```python
from build123d import *
from build123d.topology import SkipClean

# Parameters (mm, degrees)
CROQUIS1_R                      = 1.6
CROQUIS1_R_2                    = 2.75
SALIENTE_EXTRUIR1_DEPTH         = 1.5
SALIENTE_EXTRUIR3_START         = 15.1
CROQUIS3_R                      = 4
SALIENTE_EXTRUIR3_DEPTH         = 15.1
CROQUIS4_R                      = 3.1
CORTAR_EXTRUIR1_DEPTH           = 7.87
SALIENTE_EXTRUIR4_START         = -0.85
CROQUIS4_3_R                    = 3.1
CROQUIS4_3_R_2                  = 2.5
SALIENTE_EXTRUIR4_DEPTH         = 6.17
CROQUIS5_R                      = 2.5
CORTAR_EXTRUIR3_DEPTH           = 1.5
CORTAR_EXTRUIR3_DRAFT           = -17
CORTAR_EXTRUIR3_PROFILE_2_DEPTH = 1.5
CORTAR_EXTRUIR3_PROFILE_2_DRAFT = -17
CORTAR_EXTRUIR3_PROFILE_3_DEPTH = 1.5
CORTAR_EXTRUIR3_PROFILE_3_DRAFT = -17
CORTAR_EXTRUIR3_PROFILE_4_DEPTH = 1.5
CORTAR_EXTRUIR3_PROFILE_4_DRAFT = -17
NERVIO1_REACH                   = 45.809
CROQUIS6_WALL_W                 = 105.302560272
CROQUIS6_WALL_H                 = 3


with BuildPart() as part:
    # Croquis1 → Saliente-Extruir1 (new body)
    with BuildSketch(Plane(origin=(0, 0, 0), x_dir=(1, 0, 0), z_dir=(0, 1, 0))):
        with BuildLine():
            Line((-0.802944128, 3.918581469), (27.882639679, 9.796453672))
            ThreePointArc((27.882639679, 9.796453672), (39.89, 0), (27.882639679, -9.796453672))
            Line((27.882639679, -9.796453672), (-0.802944128, -3.918581469))
            ThreePointArc((-0.802944128, -3.918581469), (-4, 0), (-0.802944128, 3.918581469))
        make_face()
        with Locations(Location((29.89, 7, 0), (0, 0, 270))):
            Circle(CROQUIS1_R, mode=Mode.SUBTRACT)
        with Locations(Location((36.89, 0, 0), (0, 0, 270))):
            Circle(CROQUIS1_R, mode=Mode.SUBTRACT)
        with Locations(Location((29.89, -7, 0), (0, 0, 270))):
            Circle(CROQUIS1_R, mode=Mode.SUBTRACT)
        with Locations(Location((22.89, 0, 0), (0, 0, 270))):
            Circle(CROQUIS1_R, mode=Mode.SUBTRACT)
        with Locations(Location((29.89, 0, 0), (0, 0, 270))):
            Circle(CROQUIS1_R_2, mode=Mode.SUBTRACT)
    extrude(amount=SALIENTE_EXTRUIR1_DEPTH)

    # Croquis3 → Saliente-Extruir3 (add)
    with SkipClean():  # the faces are left unmerged after this step: merging them gives an invalid solid
        with BuildSketch(Plane.XZ.offset(SALIENTE_EXTRUIR3_START)):
            with Locations(Location((0, 0, 0), (0, 0, 258.419996521))):
                Circle(CROQUIS3_R)
        extrude(amount=-SALIENTE_EXTRUIR3_DEPTH)

    # Croquis4 → Cortar-Extruir1 (cut)
    with SkipClean():  # the faces are left unmerged after this step: merging them gives an invalid solid
        with BuildSketch(Plane.XZ.offset(15.1)):
            with Locations(Location((0, 0, 0), (0, 0, 270))):
                Circle(CROQUIS4_R)
        extrude(amount=-CORTAR_EXTRUIR1_DEPTH, mode=Mode.SUBTRACT)

    # Croquis4<3> → Saliente-Extruir4 (add)
    with SkipClean():  # the faces are left unmerged after this step: merging them gives an invalid solid
        with BuildSketch(Plane.XZ.offset(15.1).offset(SALIENTE_EXTRUIR4_START)):
            with Locations(Location((0, 0, 0), (0, 0, 270))):
                Circle(CROQUIS4_3_R)
            with Locations(Location((0, 0, 0), (0, 0, 270))):
                Circle(CROQUIS4_3_R_2, mode=Mode.SUBTRACT)
        extrude(amount=-SALIENTE_EXTRUIR4_DEPTH)


with BuildPart() as cortar_extruir3_tool:
    # Croquis5 → Cortar-Extruir3 (with draft: the straight prism first)
    with BuildSketch(Plane(origin=(0, 1.5, 0), x_dir=(1, 0, 0), z_dir=(0, 1, 0))):
        with Locations((29.89, 7)):
            Circle(CROQUIS5_R)
    extrude(amount=-CORTAR_EXTRUIR3_DEPTH)
    # Cortar-Extruir3: the draft: its side faces are tilted about the plane it starts from
    cortar_extruir3_sides = [cortar_extruir3_tool.faces().sort_by_distance(p)[0] for p in [
        (27.39, 0.75, -7),
    ]]
    draft(cortar_extruir3_sides, Plane(origin=(0, 1.5, 0), x_dir=(1, 0, 0), z_dir=(0, 1, 0)), CORTAR_EXTRUIR3_DRAFT)


with BuildPart() as part_1:
    add(part.part)

    # Cortar-Extruir3: cut by cortar_extruir3_tool
    add(cortar_extruir3_tool.part, mode=Mode.SUBTRACT)


with BuildPart() as cortar_extruir3_profile_2_tool:
    # Croquis5 → Cortar-Extruir3 profile 2 (with draft: the straight prism first)
    with BuildSketch(Plane(origin=(0, 1.5, 0), x_dir=(1, 0, 0), z_dir=(0, 1, 0))):
        with Locations((36.89, 0)):
            Circle(CROQUIS5_R)
    extrude(amount=-CORTAR_EXTRUIR3_PROFILE_2_DEPTH)
    # Cortar-Extruir3 profile 2: the draft: its side faces are tilted about the plane it starts from
    cortar_extruir3_profile_2_sides = [cortar_extruir3_profile_2_tool.faces().sort_by_distance(p)[0] for p in [
        (34.39, 0.75, 0),
    ]]
    draft(cortar_extruir3_profile_2_sides, Plane(origin=(0, 1.5, 0), x_dir=(1, 0, 0), z_dir=(0, 1, 0)), CORTAR_EXTRUIR3_PROFILE_2_DRAFT)


with BuildPart() as part_2:
    add(part_1.part)

    # Cortar-Extruir3 profile 2: cut by cortar_extruir3_profile_2_tool
    add(cortar_extruir3_profile_2_tool.part, mode=Mode.SUBTRACT)


with BuildPart() as cortar_extruir3_profile_3_tool:
    # Croquis5 → Cortar-Extruir3 profile 3 (with draft: the straight prism first)
    with BuildSketch(Plane(origin=(0, 1.5, 0), x_dir=(1, 0, 0), z_dir=(0, 1, 0))):
        with Locations((29.89, -7)):
            Circle(CROQUIS5_R)
    extrude(amount=-CORTAR_EXTRUIR3_PROFILE_3_DEPTH)
    # Cortar-Extruir3 profile 3: the draft: its side faces are tilted about the plane it starts from
    cortar_extruir3_profile_3_sides = [cortar_extruir3_profile_3_tool.faces().sort_by_distance(p)[0] for p in [
        (27.39, 0.75, 7),
    ]]
    draft(cortar_extruir3_profile_3_sides, Plane(origin=(0, 1.5, 0), x_dir=(1, 0, 0), z_dir=(0, 1, 0)), CORTAR_EXTRUIR3_PROFILE_3_DRAFT)


with BuildPart() as part_3:
    add(part_2.part)

    # Cortar-Extruir3 profile 3: cut by cortar_extruir3_profile_3_tool
    add(cortar_extruir3_profile_3_tool.part, mode=Mode.SUBTRACT)


with BuildPart() as cortar_extruir3_profile_4_tool:
    # Croquis5 → Cortar-Extruir3 profile 4 (with draft: the straight prism first)
    with BuildSketch(Plane(origin=(0, 1.5, 0), x_dir=(1, 0, 0), z_dir=(0, 1, 0))):
        with Locations((22.89, 0)):
            Circle(CROQUIS5_R)
    extrude(amount=-CORTAR_EXTRUIR3_PROFILE_4_DEPTH)
    # Cortar-Extruir3 profile 4: the draft: its side faces are tilted about the plane it starts from
    cortar_extruir3_profile_4_sides = [cortar_extruir3_profile_4_tool.faces().sort_by_distance(p)[0] for p in [
        (20.39, 0.75, 0),
    ]]
    draft(cortar_extruir3_profile_4_sides, Plane(origin=(0, 1.5, 0), x_dir=(1, 0, 0), z_dir=(0, 1, 0)), CORTAR_EXTRUIR3_PROFILE_4_DRAFT)


with BuildPart() as part_4:
    add(part_3.part)

    # Cortar-Extruir3 profile 4: cut by cortar_extruir3_profile_4_tool
    add(cortar_extruir3_profile_4_tool.part, mode=Mode.SUBTRACT)

    # Croquis6 wall → Nervio1 (add, up to next)
    with BuildSketch(Plane(origin=(10, -5.05, 0), x_dir=(-0.765076505499, -0.643939392128, 0), z_dir=(0.643939392128, -0.765076505499, 0)), mode=Mode.PRIVATE) as nervio1_sk1:
        Rectangle(CROQUIS6_WALL_W, CROQUIS6_WALL_H)
    nervio1_tool1 = extrude(nervio1_sk1.sketch, amount=-NERVIO1_REACH, mode=Mode.PRIVATE) - part_4.part
    add(nervio1_tool1.solids().sort_by_distance((10, -5.05, 0))[0])


solid = part_4.part
```
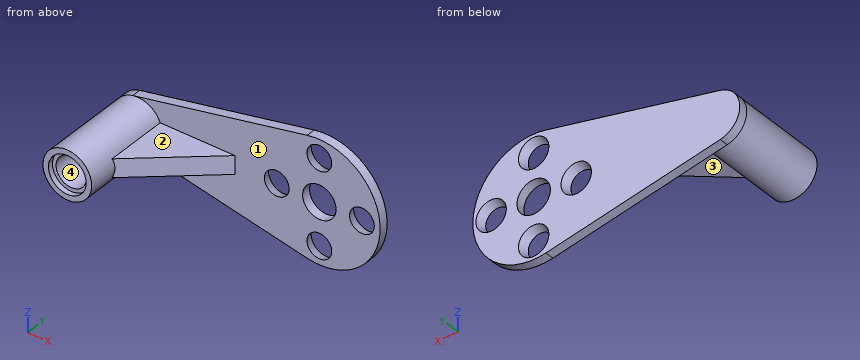
Geometry: final body of the model. Coordinates: model frame, mm. Face numbers are marked on the shaded views. Round coordinates to 2 decimals unless told otherwise and drop trailing zeros. Order: outer loops, then holes, each group sorted by start corner. A loop starts at its lowest first (then second) coordinate and runs counter-clockwise, first axis right, second up. Notation, with made-up numbers: (42.5, 40.5) -> (58.5, 40.5) arc R30 cw to (58.5, 71.5) -> close; hole circle Ø4 at (11.25, 55.25). An arc over 180 degrees is marked (long way). Use one line per item in the form item = value.
(1) Section B-B on z = -7. Return loops of the section in (x, y), and give its area (3 significant figures).
Results list:
outline = (14.24, 0) -> (27.85, 0) -> (27.39, 1.5) -> (14.24, 1.5) -> close; (31.93, 0) -> (37.03, 0) -> (37.03, 1.5) -> (32.39, 1.5) -> close
area = 27.4 mm^2
(2) Section D-D on z = 0. Count the separate pieces of the cut face and the enclosed holes in it, and give its area (3 significant figures).
Results list:
separate_pieces = 4
enclosed_holes = 0
area = 184 mm^2
(3) Draft query along Z for the marked faces 1, 2, 3 and 4. Return one class per face: pulls with the +Z half, pulls with the -Z half, needs draft (parallel to the pull), parting line crosses it, or undercut.
Results list:
face_1 = needs draft
face_2 = pulls with the +Z half
face_3 = pulls with the -Z half
face_4 = undercut
(4) Section C-C on y = -11. Return loops of the section in (x, z), and give its area (3 significant figures).
Results list:
outline = circle Ø8 at (0, 0); hole circle Ø5 at (0, 0)
area = 30.6 mm^2
(5) Section A-A on x = 22.89. Return loops of the section in (y, z), and give its area (3 significant figures).
Results list:
outline = (0, -8.77) -> (1.5, -8.77) -> (1.5, -2.5) -> (0, -2.04) -> close; (0, 2.04) -> (1.5, 2.5) -> (1.5, 8.77) -> (0, 8.77) -> close
area = 19.5 mm^2
(6) First-contact query: pin 1 Ø4.5 at (x, z) = (29.89, 0) entering from -Y; pin 2 Ø1.5 at (x, z) = (26, -5) entering from -Y; pin 3 Ø3 at (y, z) = (-7, -1) entering from +X; pin 4 Ø4.5 at (x, z) = (0, 0) entering from -Y. Flat tips, straight axial feed; report the tip coordinate or a pass-through.
Results list:
pin_1 = through
pin_2 = 0
pin_3 = 9.47
pin_4 = -7.23
(7) Ray query, probe 1 along X at (y, z) = (-10.5, 0); probe 2 along Y at (x, z) = (0.5, 3); probe 3 along X at (y, z) = (-14.65, 0). Return the intervals inside material, ascending. Write a range as [from, to].
Results list:
probe_1 = [-4, -2.5], [2.5, 4]
probe_2 = [-14.25, -8.08], [-7.23, 1.5]
probe_3 = [-4, -3.1], [3.1, 4]
